from build123d import *

# Parameters (mm, degrees)
F1_DEPTH = 6
F3_DEPTH = 0.5
F4_R     = 3
F5_DEPTH = 0.5
F6_DEPTH = 6


with BuildPart() as f1:
    # F0 (on Front) → F1 (new body)
    with BuildSketch(Plane.XZ):
        with BuildLine():
            Line((-38.911887, 40.699648), (-38.911887, 42.773143))
            ThreePointArc((-38.911887, 42.773143), (-42.363898, 40.956439), (-44.930181, 38.018585))
            ThreePointArc((-44.930181, 38.018585), (-35.761887, 21.949648), (-26.593592, 38.018585))
            ThreePointArc((-26.593592, 38.018585), (-29.159876, 40.956439), (-32.611887, 42.773143))
            Line((-32.611887, 42.773143), (-32.611887, 40.699648))
            Line((-32.611887, 40.699648), (-35.761887, 40.699648))
            Line((-35.761887, 40.699648), (-38.911887, 40.699648))
        make_face()
        with BuildLine():
            ThreePointArc((-35.761887, 35.749648), (-33.5345, 34.827035), (-32.611887, 32.599648))
            ThreePointArc((-32.611887, 32.599648), (-35.761887, 29.449648), (-38.911887, 32.599648))
            ThreePointArc((-38.911887, 32.599648), (-37.989273, 34.827035), (-35.761887, 35.749648))
        make_face(mode=Mode.SUBTRACT)
        with BuildLine():
            ThreePointArc((-44.930181, 38.018585), (-42.363898, 40.956439), (-38.911887, 42.773143))
            Line((-38.911887, 42.773143), (-38.911887, 55.949648))
            Line((-38.911887, 55.949648), (-46.411887, 51.599648))
            Line((-46.411887, 51.599648), (-46.411887, 42.599648))
            ThreePointArc((-46.411887, 42.599648), (-44.652769, 40.638466), (-44.930181, 38.018585))
        make_face()
        with BuildLine():
            ThreePointArc((-32.611887, 42.773143), (-29.159876, 40.956439), (-26.593592, 38.018585))
            ThreePointArc((-26.593592, 38.018585), (-26.871004, 40.638466), (-25.111887, 42.599648))
            Line((-25.111887, 42.599648), (-25.111887, 51.599648))
            Line((-25.111887, 51.599648), (-32.611887, 55.949648))
            Line((-32.611887, 55.949648), (-32.611887, 42.773143))
        make_face()
    extrude(amount=F1_DEPTH)

    # F2 (on face) → F3 (join)
    with BuildSketch(Plane(origin=(-32.611887, 0, 0), x_dir=(0, -1, 0), z_dir=(-1, 0, 0))):
        with BuildLine():
            ThreePointArc((3, 54.489769), (0.958263, 49.348364), (6.05872, 51.490344))
            ThreePointArc((6.05872, 51.490344), (5.159177, 53.632325), (3, 54.489769))
        make_face()
    extrude(amount=F3_DEPTH)

    # F4 (on face) → F5 (join)
    with BuildSketch(Plane.YZ.offset(-38.911887)):
        with Locations((-3.022905, 51.212981)):
            Circle(F4_R)
    extrude(amount=F5_DEPTH)

    # F0 (on Front) → F6 (join)
    with BuildSketch(Plane.XZ):
        with BuildLine():
            Line((-38.911887, 40.699648), (-38.911887, 42.773143))
            ThreePointArc((-38.911887, 42.773143), (-42.363898, 40.956439), (-44.930181, 38.018585))
            ThreePointArc((-44.930181, 38.018585), (-35.761887, 21.949648), (-26.593592, 38.018585))
            ThreePointArc((-26.593592, 38.018585), (-29.159876, 40.956439), (-32.611887, 42.773143))
            Line((-32.611887, 42.773143), (-32.611887, 40.699648))
            Line((-32.611887, 40.699648), (-35.761887, 40.699648))
            Line((-35.761887, 40.699648), (-38.911887, 40.699648))
        make_face()
        with BuildLine():
            ThreePointArc((-35.761887, 35.749648), (-33.5345, 34.827035), (-32.611887, 32.599648))
            ThreePointArc((-32.611887, 32.599648), (-35.761887, 29.449648), (-38.911887, 32.599648))
            ThreePointArc((-38.911887, 32.599648), (-37.989273, 34.827035), (-35.761887, 35.749648))
        make_face(mode=Mode.SUBTRACT)
        with BuildLine():
            ThreePointArc((-44.930181, 38.018585), (-42.363898, 40.956439), (-38.911887, 42.773143))
            Line((-38.911887, 42.773143), (-38.911887, 55.949648))
            Line((-38.911887, 55.949648), (-46.411887, 51.599648))
            Line((-46.411887, 51.599648), (-46.411887, 42.599648))
            ThreePointArc((-46.411887, 42.599648), (-44.652769, 40.638466), (-44.930181, 38.018585))
        make_face()
        with BuildLine():
            ThreePointArc((-32.611887, 42.773143), (-29.159876, 40.956439), (-26.593592, 38.018585))
            ThreePointArc((-26.593592, 38.018585), (-26.871004, 40.638466), (-25.111887, 42.599648))
            Line((-25.111887, 42.599648), (-25.111887, 51.599648))
            Line((-25.111887, 51.599648), (-32.611887, 55.949648))
            Line((-32.611887, 55.949648), (-32.611887, 42.773143))
        make_face()
    extrude(amount=F6_DEPTH)


solid = f1.part
For this review, take the finished solid that the model builds, in its own axes (mm). A direction names the side the tool comes from. Round coordinates to 2 decimals unless told otherwise and drop trailing zeros. Loops run counter-clockwise (first coordinate to the right, second up) from the corner with the lowest first, then second, coordinate; pieces in that order, holes last. Notation, with made-up numbers: (-13.5, -7) - (22.5, -7) arc R31 ccw to (22.5, 32) - close; hole circle Ø3 at (57.5, 15.25). An arc over 180 degrees is marked (long way). Put each result on its own line as item: value. Start each with the question number.
1. Consider section B-B on x = -35.25. State the section outline as (y, z) points.
2. Insertion check: P1, Ø8, axis at x = -35, z = 28, coming from the -Y side; P2, Ø1, axis at x = -37.5, y = -2.5, coming from the +Z side; P3, Ø3, axis at y = -1.5, z = 25.5, coming from the +X side. Each pin has a flat end and moves straight along its axis. Give the tip position at first contact, or say it passes through.
3. Mouldability with a two-part tool opening along X and no side actions: class faces 1 (the flat face through (-36, 0, 39)), 2 (the flat face through (-38.912, -3, 47)), 3 (the cylindrical face through (-36.076, -2.958, 21.954)), 4 (the cylindrical face through (-44.665, -2.958, 40.675)) as +X half, -X half, draft (parallel to the pull), parting line (faces both ways), or undercut.
4. Consider section A-A on z = 43. State the section outline as (x, y) points.
5. Consider section C-C on y = -2. State the section outline as (x, z) points.
6. For faces 5 (the cylindrical face through (-38.665, -5.234, 53.241)), 6 (the flat face through (-25.112, -3, 47)), list the 3-axis set-ups (+Z, -Z, +X, -X, +Y, -Y) from which the entire face can be reached by the end or side of a thin tool; tool diameter is ignored.
7. Consider section D-D on x = -28.5. State the section outline as (y, z) points.
8. For probe 1 along X at (y, z) = (-1.5, 46); probe 2 along Y at (x, z) = (-38.5, 26); probe 3 along X at (y, z) = (-4.25, 35), list the stretches that pass through material, from the lowest coordinate up. Write a range as [from, to].
Result sheet:
1. outline: (-6, 21.96) - (0, 21.96) - (0, 29.49) - (-6, 29.49) - close; (-6, 35.71) - (0, 35.71) - (0, 40.7) - (-6, 40.7) - close
2. P1: y = -6
2. P2: z = 40.7
2. P3: x = -26.7
3. face 1: draft
3. face 2: undercut
3. face 3: parting line
3. face 4: -X half
4. outline: (-46.41, -6) - (-38.91, -6) - (-38.91, 0) - (-46.41, 0) - close; (-32.61, -6) - (-25.11, -6) - (-25.11, 0) - (-32.61, 0) - close
5. outline: (-46.41, 42.6) arc R3.24 cw to (-44.93, 38.02) arc R10.65 ccw (long way) to (-26.59, 38.02) arc R3.24 cw to (-25.11, 42.6) - (-25.11, 51.6) - (-32.61, 55.95) - (-32.61, 54.3) - (-33.11, 54.3) - (-33.11, 48.68) - (-32.61, 48.68) - (-32.61, 40.7) - (-38.91, 40.7) - (-38.91, 48.39) - (-38.41, 48.39) - (-38.41, 54.03) - (-38.91, 54.03) - (-38.91, 55.95) - (-46.41, 51.6) - close; hole (-35.76, 35.75) arc R3.15 ccw (long way) to (-32.61, 32.6) arc R3.15 ccw to start
6. face 5: none
6. face 6: +Z, -Z, +X, +Y, -Y
7. outline: (-6, 24.81) - (0, 24.81) - (0, 53.56) - (-6, 53.56) - close
8. probe 1: [-46.41, -38.91], [-32.61, -25.11]
8. probe 2: [-6, 0]
8. probe 3: [-46.14, -37.8], [-33.72, -25.39]
